Autodesk Inventor part; units mm, degrees
ref_plane "YZ Plane" through (0, 0, 0) normal (1, 0, 0) x (0, 1, 0)
ref_plane "XZ Plane" through (0, 0, 0) normal (0, 1, 0) x (-1, 0, 0)
ref_plane "XY Plane" through (0, 0, 0) normal (0, 0, 1) x (1, 0, 0)
sketch "Sketch_1" plane through (0, 0, 0) normal (0, 0, 1) x (1, 0, 0)
  line L0 (0, 22) -> (0, 4)
  line L1 (0, 4) -> (15, 4)
  line L2 (15, 4) -> (15, 22)
  arc A0 (15, 22) -> (13, 24) centre (13, 22) ccw
  line L3 (13, 24) -> (2, 24)
  arc A1 (2, 24) -> (0, 22) centre (2, 22) ccw
extrude "Extrusion1" add sketch "Sketch_1" against normal blind 12
sketch "Sketch_8" plane through (6.5, 0, 0) normal (1, 0, 0) x (0, 0, -1)
  line L0 (0, 16) -> (12, 16)
  line L1 (12, 16) -> (12, 13)
  line L2 (12, 13) -> (11.5, 13.5)
  line L3 (11.5, 13.5) -> (0.5, 13.5)
  line L4 (0.5, 13.5) -> (0, 13)
  line L5 (0, 13) -> (0, 16)
  line L6 (0, 16) -> (12, 16)
revolve "Revolution1" cut sketch "Sketch_8" angle 360 about axis through (6.5, 16, 0) along (0, 0, 1)
sketch "Sketch_9" plane through (8.5, 0, 0) normal (1, 0, 0) x (0, 0, -1)
  line L0 (0, 16) -> (12, 16)
  line L1 (12, 16) -> (12, 13)
  line L2 (12, 13) -> (11.5, 13.5)
  line L3 (11.5, 13.5) -> (0.5, 13.5)
  line L4 (0.5, 13.5) -> (0, 13)
  line L5 (0, 13) -> (0, 16)
  line L6 (0, 16) -> (12, 16)
revolve "Revolution2" cut sketch "Sketch_9" angle 360 about axis through (8.5, 16, 0) along (0, 0, 1)
sketch "Sketch_10" plane through (6.5, 0, 0) normal (1, 0, 0) x (0, 0, -1)
  line L0 (0, 13) -> (0.5, 13.5)
  line L1 (0.5, 13.5) -> (11.5, 13.5)
  line L2 (11.5, 13.5) -> (12, 13)
  line L3 (12, 13) -> (12, 19)
  line L4 (12, 19) -> (11.5, 18.5)
  line L5 (11.5, 18.5) -> (0.5, 18.5)
  line L6 (0.5, 18.5) -> (0, 19)
  line L7 (0, 19) -> (0, 13)
extrude "Extrusion2" cut sketch "Sketch_10" along normal blind 2
sketch "Sketch_7" plane through (7.5, 0, 0) normal (1, 0, 0) x (0, 0, -1)
  line L0 (-0.5, 1.15) -> (2.1, -0.3)
  line L1 (2.1, -0.3) -> (7.9, -0.3)
  line L2 (7.9, -0.3) -> (10.5, 1.15)
  line L3 (10.5, 1.15) -> (10.5, 2.5)
  line L4 (10.5, 2.5) -> (7.9, 2.5)
  line L5 (7.9, 2.5) -> (7.9, 4)
  line L6 (7.9, 4) -> (2.1, 4)
  line L7 (2.1, 4) -> (2.1, 2.5)
  line L8 (2.1, 2.5) -> (-0.5, 2.5)
  line L9 (-0.5, 2.5) -> (-0.5, 1.15)
sketch "Sketch_3" plane through (0, 0, 0) normal (1, 0, 0) x (0, 1, 0)
  line L0 (6.2, -2) -> (6.2, -5)
  line L1 (6.2, -5) -> (9.45, -5)
  line L2 (9.45, -5) -> (9.45, -2)
  line L3 (9.45, -2) -> (6.2, -2)
sketch "Sketch_5" plane through (0, 0, 0) normal (1, 0, 0) x (0, 1, 0)
  line L0 (6.2, -7) -> (6.2, -10)
  line L1 (6.2, -10) -> (9.45, -10)
  line L2 (9.45, -10) -> (9.45, -7)
  line L3 (9.45, -7) -> (6.2, -7)
extrude "Extrusion3" cut sketch "Sketch_3" along normal blind 15
extrude "Extrusion4" cut sketch "Sketch_5" along normal blind 15
sketch "Sketch_6" plane through (0, 0, 0) normal (0, 0, 1) x (1, 0, 0)
  line L0 (2, 6.2) -> (13, 6.2)
  line L1 (13, 6.2) -> (13, 9.45)
  line L2 (13, 9.45) -> (2, 9.45)
  line L3 (2, 9.45) -> (2, 6.2)
extrude "Extrusion5" cut sketch "Sketch_6" against normal blind 0.5
sketch "Sketch_11" plane through (0, 0, 0) normal (0, 1, 0) x (-1, 0, 0)
  line L0 (-7.2, 0) -> (-7.8, 0)
  line L1 (-7.8, 0) -> (-7.5, -0.3)
  line L2 (-7.5, -0.3) -> (-7.2, 0)
extrude "Extrusion6" cut sketch "Sketch_11" along normal blind 25
sketch "Sketch_12" plane through (0, 0, 0) normal (0, 1, 0) x (-1, 0, 0)
  line L0 (-7.2, -12) -> (-7.5, -11.7)
  line L1 (-7.5, -11.7) -> (-7.8, -12)
  line L2 (-7.8, -12) -> (-7.2, -12)
extrude "Extrusion7" cut sketch "Sketch_12" along normal blind 25
extrude "Extrusion8" add sketch "Sketch_7" along normal mid plane 5.4
sketch "Sketch_2" plane through (7.5, 0, 0) normal (1, 0, 0) x (0, 0, -1)
  line L0 (5, -0.3) -> (5, -1.3)
  line L1 (5, -1.3) -> (3.364, -1.3)
  line L2 (3.364, -1.3) -> (3, -0.3)
  line L3 (3, -0.3) -> (5, -0.3)
  line L4 (5, -0.3) -> (5, -1.3)
revolve "Revolution3" add sketch "Sketch_2" angle 360 about axis through (7.5, -0.3, -5) along (0, 1, 0)
sketch "Sketch_4" plane through (0, 0, 0) normal (0, 1, 0) x (-1, 0, 0)
  line L0 (-3.8, 1.5) -> (-10.2, 1.5)
  line L1 (-10.2, 1.5) -> (-10.2, 0.5)
  line L2 (-10.2, 0.5) -> (-8.7, 0.5)
  arc A0 (-4.8, -1.5) -> (-8.7, 0.5) centre (-8.8008, -4.499) ccw
  line L3 (-4.8, -1.5) -> (-3.8, -1.5)
  line L4 (-3.8, -1.5) -> (-3.8, 1.5)
extrude "Extrusion9" cut sketch "Sketch_4" along normal blind 3
sketch "Sketch_13" plane through (0, 0, 0) normal (0, 1, 0) x (-1, 0, 0)
  line L0 (-4.8, -10.5) -> (-6.3, -10.5)
  arc A0 (-10.2, -8.5) -> (-6.3, -10.5) centre (-6.1992, -5.501) ccw
  line L1 (-10.2, -8.5) -> (-11.2, -8.5)
  line L2 (-11.2, -8.5) -> (-11.2, -11.5)
  line L3 (-11.2, -11.5) -> (-4.8, -11.5)
  line L4 (-4.8, -11.5) -> (-4.8, -10.5)
extrude "Extrusion10" cut sketch "Sketch_13" along normal blind 3
sketch "Sketch_14" plane through (10.2, 0, 0) normal (1, 0, 0) x (0, 0, -1)
  circle A0 centre (5, 1.5) radius 0.7
extrude "Extrusion11" cut sketch "Sketch_14" against normal blind 0.3
sketch "Sketch_15" plane through (0, 0, -0.5) normal (0, 0, 1) x (1, 0, 0)
  arc A0 (6.5, 18.5) -> (6.5, 13.5) centre (6.5, 16) ccw
  line L0 (6.5, 13.5) -> (8.5, 13.5)
  arc A1 (8.5, 13.5) -> (8.5, 18.5) centre (8.5, 16) ccw
  line L1 (8.5, 18.5) -> (6.5, 18.5)
extrude "Extrusion12" add sketch "Sketch_15" against normal blind 11
sketch "Sketch_16" plane through (7.5, 0, 0) normal (1, 0, 0) x (0, 0, -1)
  line L0 (0.5, 16) -> (11.5, 16)
  line L1 (11.5, 16) -> (11.5, 13.5)
  line L2 (11.5, 13.5) -> (11.067, 13.933)
  line L3 (11.067, 13.933) -> (0.933, 13.933)
  line L4 (0.933, 13.933) -> (0.5, 13.5)
  line L5 (0.5, 13.5) -> (0.5, 16)
  line L6 (0.5, 16) -> (11.5, 16)
revolve "Revolution4" cut sketch "Sketch_16" angle 360 about axis through (7.5, 16, -0.5) along (0, 0, 1)
thread "Thread1"
sketch "Sketch_17" plane through (0, 4, 0) normal (0, 1, 0) x (1, 0, 0)
  line L0 (2, 10) -> (2, 0)
  line L1 (2, 0) -> (12, 0)
  line L2 (12, 0) -> (12, 10)
  line L3 (12, 10) -> (2, 10)
  line L4 (4.8, 3.0522) -> (10.2, 2.1)
  line L5 (10.2, 2.1) -> (10.2, 6.9478)
  line L6 (10.2, 6.9478) -> (4.8, 7.9)
  line L7 (4.8, 7.9) -> (4.8, 3.0522)
extrude "Extrusion13" cut sketch "Sketch_17" against normal blind 1.5
sketch "Sketch_18" plane through (0, 2.5, 0) normal (0, 1, 0) x (1, 0, 0)
  line L0 (11.7, 15) -> (11.7, -5)
  line L1 (2.8, 3.4048) -> (2.8, -5)
  line L2 (2.8, -5) -> (11.2, -5)
  line L3 (11.2, -5) -> (11.2, 1.9237)
  line L4 (11.2, 1.9237) -> (2.8, 3.4048)
revolve "Revolution5" cut sketch "Sketch_18" angle 10 about axis through (11.7, 2.5, -15) along (0, 0, 1)
sketch "Sketch_19" plane through (0, 2.5, 0) normal (0, 1, 0) x (1, 0, 0)
  line L0 (3.3, -5) -> (3.3, 15)
  line L1 (3.8, 8.0763) -> (12.2, 6.5952)
  line L2 (12.2, 6.5952) -> (12.2, 15)
  line L3 (12.2, 15) -> (3.8, 15)
  line L4 (3.8, 15) -> (3.8, 8.0763)
revolve "Revolution6" cut sketch "Sketch_19" angle 10 about axis through (3.3, 2.5, 5) along (0, 0, -1)
properties part number "HCBR5"
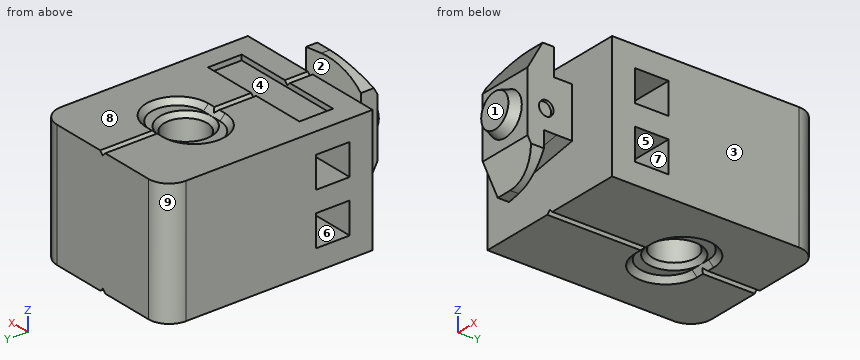
The model under review builds one solid part; all positions refer to its coordinate system, in mm. Face numbers are marked on the shaded views. A direction names the side the tool comes from. Give positions to 0.01 mm unless a question says otherwise; leave off trailing zeros. Write each loop counter-clockwise with the first axis right and the second up, starting at its lowest first coordinate (ties: lowest second). Pieces come first, ordered by that corner, then holes. Notation, with made-up numbers: M 64,73 L 107,73 A11 cw 107,92 Z; hole C 31.25,85.5 d10. An arc over 180 degrees is marked long. Answer in a Markdown table with one row per item.
Item 1: Add section A-A on x = 13.5. Give the boundary of the cut face in (y, z).
Check sheet entries:
| item | result |
|---|---|
| outline | M 4,-12 L 23.94,-12 L 23.94,0 L 4,0 Z; hole M 6.2,-10 L 9.45,-10 L 9.45,-7 L 6.2,-7 Z; hole M 6.2,-5 L 9.45,-5 L 9.45,-2 L 6.2,-2 Z |
Item 2: Tool access review of the marked faces 1, 2, 3, 4 and 5: name each direction out of +Z, -Z, +X, -X, +Y, -Y from which nothing blocks a thin tool from reaching the whole face with its end or side.
Check sheet entries:
| item | result |
|---|---|
| face 1 | +Z, -Z, +X, -X, -Y |
| face 2 | +Z, -X |
| face 3 | +Z, -Z, +X, +Y, -Y |
| face 4 | +Z |
| face 5 | +X, -X |
Item 3: For P1, Ø1.8, axis at x = 6.5, y = 16, coming from the +Z side; P2, Ø5, axis at x = 11.5, z = -2.5, coming from the -Y side; P3, Ø2, axis at x = 13, y = 13, coming from the +Z side; P4, Ø1.1, axis at y = 1.5, z = -5, coming from the -X side, all flat-tipped, find the tip position at first contact; note any pin that passes through.
Check sheet entries:
| item | result |
|---|---|
| P1 | through |
| P2 | y = -0.3 |
| P3 | z = 0 |
| P4 | x = 4.8 |
Item 4: Draft analysis for pull direction Y (two halves, no side actions). For the marked faces 6, 7, 8 and 9, state which applies: +Y half, -Y half, draft (parallel to the pull), parting line (faces both ways), or undercut.
Check sheet entries:
| item | result |
|---|---|
| face 6 | undercut |
| face 7 | undercut |
| face 8 | draft |
| face 9 | +Y half |
Item 5: For line 1 along Z through (x, y) = (4, 7.75); line 2 along Y through (x, z) = (12.75, -3.5); line 3 along X through (y, z) = (16, -3.5), list the stretches that pass through material, from the lowest coordinate up.
Check sheet entries:
| item | result |
|---|---|
| line 1 | -12 to -10, -7 to -5, -2 to -0.5 |
| line 2 | 4 to 6.2, 9.45 to 24 |
| line 3 | 0 to 5.43, 9.57 to 15 |
